from build123d import *

# Parameters (mm, degrees)
F2_R     = 10.9427513267
F6_DEPTH = 12.7


# Not quite as in the source:
# - a feature of the source that left no trace in its solid (it failed there, or was rolled back) is left out


with BuildPart() as f1:
    # F0 (on Top) → F1 (revolve)
    with BuildSketch(Plane.XY):
        Polygon((-22.4952585995, 7.654638961), (-22.4952585995, 0), (0, 0), (0, 51.6905076802), (-22.4952585995, 10.4665467516), (-5.6238141842, 10.4665467516), (-5.6238141842, 7.654638961), align=None)
        Polygon((-22.4952585995, 0), (-33.1180207431, 0), (-33.1180207431, -5.9848567471), (0, -5.9848567471), (0, 0), align=None)
    revolve(axis=Axis((0, -2.9924283735, 0), (0, -1, 0)))

    # F4: sweep along a path in F3
    with BuildLine(Plane.XY) as f4_path:
        Line((0, -6.7567974329), (0, -50.1213520765))
    # F2 (on face) → F4 (sweep)
    with BuildSketch(Plane.XZ.offset(5.9848567471)):
        Circle(F2_R)
    sweep(path=f4_path.line)

    # F5 (on face) → F6 (join)
    with BuildSketch(Plane.XZ.offset(5.9848567471)):
        with BuildLine():
            ThreePointArc((0, 25.6462656645), (-18.1346483635, -18.1346483635), (25.6462656645, 0))
            ThreePointArc((25.6462656645, 0), (18.1346483635, 18.1346483635), (0, 25.6462656645))
        make_face()
        with BuildLine():
            ThreePointArc((-10.2304533567, 3.8835075273), (-6.214802871, 9.0066659687), (0, 10.9427513267))
            ThreePointArc((0, 10.9427513267), (6.3686758751, 8.8985265182), (10.3578760896, 3.5296188901))
            ThreePointArc((10.3578760896, 3.5296188901), (10.7955423421, 1.7888745451), (10.9427513267, 0))
            ThreePointArc((10.9427513267, 0), (9.4510721789, -5.5155272882), (5.3827161292, -9.5273382259))
            ThreePointArc((5.3827161292, -9.5273382259), (0, -10.9427513267), (-5.3827161292, -9.5273382259))
            ThreePointArc((-5.3827161292, -9.5273382259), (-10.2910379118, -3.7199926472), (-10.2304533567, 3.8835075273))
        make_face(mode=Mode.SUBTRACT)
    extrude(amount=F6_DEPTH)


solid = f1.part
Model file for the job. Use its own axes, mm. A direction names the side the tool comes from. Give positions to 0.01 mm unless a question says otherwise; leave off trailing zeros. Order: outer loops, then holes, each group sorted by start corner. A loop starts at its lowest first (then second) coordinate and runs counter-clockwise, first axis right, second up. Notation, with made-up numbers: (27.5, -24) -> (62.5, -24) arc R14 ccw to (62.5, -20) -> close; hole circle Ø6 at (-38, 13). An arc over 180 degrees is marked (long way). Use CSV: the item, a comma, the result in double quotes.
1. Drill centre lines: line 1 along Y through (x, z) = (0.5, -28.5); line 2 along X through (y, z) = (-29, 0); line 3 along Y through (x, z) = (-3, 6.5). Where is each one in solid material? Low to high. Write a range as from..to.
Outcome:
line 1,"-5.98..0"
line 2,"-10.94..10.94"
line 3,"-49.35..7.65, 10.47..38.57"
2. 3-axis set-ups, long thin cutter, end or side, ignore diameter. For faces 5 (the flat face through (5, -18.685, -11)), 6 (the flat face through (-5, 10.467, 5)), 7 (the flat face through (0, -49.349, 0)), 8 (the cylindrical face through (-21.456, 3.774, -6.757)): which of +Z, -Z, +X, -X, +Y, -Y reach the whole face in a straight line?
Outcome:
face 5,"-Y"
face 6,"none"
face 7,"+Z, -Z, +X, -X, -Y"
face 8,"+Y"
3. Band-saw the part on B-B, the plane y = 34. Give the cut face in (x, z).
Outcome:
outline,"circle Ø19.31 at (0, 0)"
4. Band-saw the part on A-A, the plane x = 24. Give the cut face in (y, z), then the cut area to 3 significant figures.
Outcome:
outline,"(-18.68, -9.04) -> (-5.98, -9.04) -> (-5.98, -22.82) -> (0, -22.82) -> (0, 22.82) -> (-5.98, 22.82) -> (-5.98, 9.04) -> (-18.68, 9.04) -> close"
area,"503 mm²"
5. Drop flat-ended pins along their axis: pin 1 (10 mm diameter, centred on y = 6.5, z = 6, fed in from +X); pin 2 (1 mm diameter, centred on x = 17, y = -5.5, fed in from +Z); pin 3 (6 mm diameter, centred on y = -30, z = -5.5, fed in from -X). Give the stop position or say it passes through.
Outcome:
pin 1,"x = 22.47"
pin 2,"z = 28.72"
pin 3,"x = -10.65"
6. Mould opens along Y. For faces 1 (the flat face through (-17, -5.985, 19.5)), 2 (the flat face through (5, 7.655, 5)), 3 (the cylindrical face through (24.41, -3.03, -22.38)), 4 (the flat face through (22, 0, 7)) say: +Y half, -Y half, draft (parallel to the pull), parting line (faces both ways), or undercut.
Outcome:
face 1,"-Y half"
face 2,"undercut"
face 3,"draft"
face 4,"+Y half"
7. Band-saw the part on C-C, the plane y = 21. Give the cut face in (x, z), then the cut area to 3 significant figures.
Outcome:
outline,"circle Ø33.49 at (0, 0)"
area,"881 mm²"
